Autodesk Inventor part; units mm, degrees
ref_plane "YZ Plane" through (0, 0, 0) normal (1, 0, 0) x (0, 1, 0)
ref_plane "XZ Plane" through (0, 0, 0) normal (0, 1, 0) x (-1, 0, 0)
ref_plane "XY Plane" through (0, 0, 0) normal (0, 0, 1) x (1, 0, 0)
sketch "Sketch1" plane through (0, 0, 0) normal (0, 0, 1) x (1, 0, 0)
  line L0 (0, 0) -> (25.4, 0)
  line L1 (25.4, 0) -> (25.4, 25.4)
  line L2 (25.4, 25.4) -> (0, 25.4)
  line L3 (0, 25.4) -> (0, 0)
  dimension "d0" = 25.4
  dimension "d1" = 25.4
extrude "Extrusion1" add sketch "Sketch1" along normal blind 406.4
shell "Shell1" thickness 1.5875 removed faces 2 at (8.4667, 16.9333, 0) at (8.4667, 16.9333, 406.4)
sketch "Sketch2" plane through (25.4, 0, 0) normal (1, 0, 0) x (0, 0, -1)
  line L0 (-406.4, 25.4) -> (-406.4, 0)
  line L1 (0, 25.4) -> (-406.4, 25.4)
  circle A0 centre (-393.7, 12.7) radius 2.3813
  dimension "d5" = 4.7625
  dimension "d6" = 12.7
  dimension "d7" = 12.7
extrude "Extrusion2" cut sketch "Sketch2" against normal through all
pattern_linear "Rectangular Pattern1" count 16 spacing 25.4 along (0, 0, -1) of "Extrusion2"
properties part number "Frame_TopRail" material "Aluminum-6061"
Work out the finished part from the listing and answer in its coordinate system (mm). A direction names the side the tool comes from. Round coordinates to 2 decimals unless told otherwise and drop trailing zeros. Write each loop counter-clockwise with the first axis right and the second up, starting at its lowest first coordinate (ties: lowest second). Pieces come first, ordered by that corner, then holes.
1) A cutting plane is placed at C-C on z = 302. Determine the outline of the cut face in (x, y).
2) Determine the mould class of faces 1 (the face through (13, 0, 200)), 2 (the face through (1.588, 13, 200)), 3 (the face through (25.4, 13, 200)) for opening direction Y: pulls with the +Y half, pulls with the -Y half, needs draft (parallel to the pull), parting line crosses it, or undercut.
3) Consider probe 1 along X at (y, z) = (5, 250); probe 2 along Y at (x, z) = (24.3, 266.7). Determine where each line is inside the solid, lowest interval first.
4) A flat-ended cylindrical pin translates along its axis: P1, Ø3, axis at y = 12.7, z = 63.5, coming from the -X side. Find the tip coordinate at first contact, or state that the pin passes through.
5) Which of the six approach directions +Z, -Z, +X, -X, +Y, -Y give full straight-line access (tool end or side, diameter ignored) to faces 4 (the face through (13, 25.4, 200)), 5 (the face through (13, 1.588, 200))?
6) A cutting plane is placed at A-A on y = 20.5. Determine the outline of the cut face in (x, z).
Entries:
1. outline: (0, 0) - (25.4, 0) - (25.4, 25.4) - (0, 25.4) - close; hole (1.59, 1.59) - (23.81, 1.59) - (23.81, 23.81) - (1.59, 23.81) - close
2. face 1: pulls with the -Y half
2. face 2: undercut
2. face 3: needs draft
3. probe 1: x = 0 to 1.59, 23.81 to 25.4
3. probe 2: y = 0 to 10.32, 15.08 to 25.4
4. P1: passes through
5. face 4: +Z, -Z, +X, -X, +Y
5. face 5: +Z, -Z
6. outline: (0, 0) - (1.59, 0) - (1.59, 406.4) - (0, 406.4) - close; (23.81, 0) - (25.4, 0) - (25.4, 406.4) - (23.81, 406.4) - close
